```python
from build123d import *

# Parameters (mm, degrees)
SKETCH1_W           = 294
SKETCH1_H           = 210
BOSS_EXTRUDE1_DEPTH = 18.5
CUT_EXTRUDE1_DEPTH  = 300
CHAMFER1_SIZE       = 6
CHAMFER1_SIZE2      = 10.392304845
FILLET1_R           = 40
FILLET2_R           = 4
FILLET3_R           = 50
SKETCH3_W           = 6.7
SKETCH3_H           = 10
BOSS_EXTRUDE2_DEPTH = 11
FILLET4_R           = 5
SKETCH4_W           = 284
SKETCH4_H           = 123.889727457
BOSS_EXTRUDE3_DEPTH = 2


with BuildPart() as part:
    # Sketch1 → Boss-Extrude1 (new body)
    with BuildSketch(Plane(origin=(0, 0, 0), x_dir=(1, 0, 0), z_dir=(0, 1, 0))):
        Rectangle(SKETCH1_W, SKETCH1_H)
    extrude(amount=BOSS_EXTRUDE1_DEPTH)

    # Sketch2 → Cut-Extrude1 (cut)
    with BuildSketch(Plane(origin=(147, 0, 0), x_dir=(0, 0, -1), z_dir=(1, 0, 0))):
        Polygon((-105, 6.5), (-65, 0), (-105, 0), align=None)
    extrude(amount=-CUT_EXTRUDE1_DEPTH, mode=Mode.SUBTRACT)

    # Chamfer1
    chamfer1_edges = [part.edges().sort_by_distance(p)[0] for p in [
        (0, 18.5, 105),
    ]]
    chamfer1_side = [part.faces().sort_by_distance(p)[0] for p in [
        (0, 12.5, 105),
    ]]
    chamfer(chamfer1_edges, length=CHAMFER1_SIZE, length2=CHAMFER1_SIZE2, reference=chamfer1_side[0])

    # Fillet1
    fillet1_edges = [part.edges().sort_by_distance(p)[0] for p in [
        (0, 18.5, 94.607695155),
    ]]
    fillet(fillet1_edges, radius=FILLET1_R)

    # Fillet2
    fillet2_edges = [part.edges().sort_by_distance(p)[0] for p in [
        (0, 6.5, 105),
        (0, 12.5, 105),
    ]]
    fillet(fillet2_edges, radius=FILLET2_R)

    # Fillet3
    fillet3_edges = [part.edges().sort_by_distance(p)[0] for p in [
        (0, 0, 65),
    ]]
    fillet(fillet3_edges, radius=FILLET3_R)

    # Sketch3 → Boss-Extrude2 (add)
    with BuildSketch(Plane(origin=(0, 18.5, 0), x_dir=(1, 0, 0), z_dir=(0, 1, 0))):
        with Locations((128.65, 100)):
            Rectangle(SKETCH3_W, SKETCH3_H)
        with Locations((-128.65, 100)):
            Rectangle(SKETCH3_W, SKETCH3_H)
    extrude(amount=BOSS_EXTRUDE2_DEPTH)

    # Fillet4
    fillet4_edges = [part.edges().sort_by_distance(p)[0] for p in [
        (128.65, 29.5, -105),
        (128.65, 29.5, -95),
        (-128.65, 29.5, -105),
        (-128.65, 29.5, -95),
    ]]
    fillet(fillet4_edges, radius=FILLET4_R - 0.0001)  # a hair under: the kernel refuses the full size

    # Sketch4 → Boss-Extrude3 (add)
    with BuildSketch(Plane(origin=(0, 18.5, 0), x_dir=(1, 0, 0), z_dir=(0, 1, 0))):
        with Locations((0, 23.055136272)):
            Rectangle(SKETCH4_W, SKETCH4_H)
    extrude(amount=BOSS_EXTRUDE3_DEPTH)


solid = part.part
```
The model under review builds one solid part; all positions refer to its coordinate system, in mm. A direction names the side the tool comes from. Coordinates: 2 decimals unless noted, no trailing zeros. Write each loop counter-clockwise with the first axis right and the second up, starting at its lowest first coordinate (ties: lowest second). Pieces come first, ordered by that corner, then holes. Notation, with made-up numbers: (0, 65.25) - (33, 65.25) arc R20 ccw to (33, 102.25) - close; hole circle Ø4 at (74.5, -32.5). An arc over 180 degrees is marked (long way). Answer in a Markdown table with one row per item. Add a question column.
Q1. Draft analysis for pull direction Z (two halves, no side actions). For faces 1 (the face through (129, 21, -95)), 2 (the face through (-125.3, 24, -100)), 3 (the face through (-2.058, 0.158, 64.931)), state which applies: +Z half, -Z half, draft (parallel to the pull), parting line (faces both ways), or undercut.
Q2. To check wall thickness, follow line 1 along X through (y, z) = (20.25, -43.5); line 2 along Y through (x, z) = (-70, -68.5); line 3 along Y through (x, z) = (32.5, 53.5). State the ranges of each line that lie inside material, in increasing order. Write a range as from..to.
Q3. Consider section A-A on z = -29. Give the boundary of the cut face in (x, y).
Q4. For faces 4 (the face through (-129, 21, -95)), 5 (the face through (125.3, 24, -100)), 6 (the face through (-132, 24, -100)), list the 3-axis set-ups (+Z, -Z, +X, -X, +Y, -Y) from which the entire face can be reached by the end or side of a thin tool; tool diameter is ignored.
Q5. Clearance check with flat-ended pins moving along their axes: pin 1 (5 mm diameter, centred on y = 23.5, z = -99.5, fed in from +X); pin 2 (3 mm diameter, centred on y = 21.5, z = -101.5, fed in from -X); pin 3 (1.8 mm diameter, centred on x = 127.5, y = 20.5, fed in from +Z); pin 4 (1 mm diameter, centred on x = 83.5, y = 21.5, fed in from +Z). State where each tip first meets the part, or that it passes through.
Answers below:
| question | item | result |
|---|---|---|
| 1 | face 1 | undercut |
| 1 | face 2 | draft |
| 1 | face 3 | +Z half |
| 2 | line 1 | -142..142 |
| 2 | line 2 | 0..20.5 |
| 2 | line 3 | 0..18.5 |
| 3 | outline | (-147, 0) - (147, 0) - (147, 18.5) - (142, 18.5) - (142, 20.5) - (-142, 20.5) - (-142, 18.5) - (-147, 18.5) - close |
| 4 | face 4 | +X, -X, +Y |
| 4 | face 5 | -Z, +Y |
| 4 | face 6 | -Z, -X, +Y |
| 5 | pin 1 | x = 132 |
| 5 | pin 2 | x = -132 |
| 5 | pin 3 | z = 38.89 |
| 5 | pin 4 | through |
